Autodesk Inventor part; units mm, degrees
ref_plane "YZ Plane" through (0, 0, 0) normal (1, 0, 0) x (0, 1, 0)
ref_plane "XZ Plane" through (0, 0, 0) normal (0, 1, 0) x (-1, 0, 0)
ref_plane "XY Plane" through (0, 0, 0) normal (0, 0, 1) x (1, 0, 0)
sketch "Эскиз1" plane through (0, 0, 0) normal (0, 1, 0) x (-1, 0, 0)
  line L0 (-150, 150) -> (150, 150)
  line L1 (150, 150) -> (150, -150)
  line L2 (150, -150) -> (-150, -150)
  line L3 (-150, -150) -> (-150, 150)
  line L4 (-150, 150) -> (150, -150) construction
  line L5 (150, 150) -> (-150, -150) construction
  circle A0 centre (125, -125) radius 8.5
  circle A1 centre (0, -125) radius 8.5
  circle A2 centre (-125, -125) radius 8.5
  circle A3 centre (125, 125) radius 8.5
  circle A4 centre (0, 125) radius 8.5
  circle A5 centre (40, 100) radius 8.5
  circle A6 centre (40, 65) radius 8.5
  circle A7 centre (40, 30) radius 8.5
  circle A8 centre (-40, 30) radius 8.5
  circle A9 centre (-40, 65) radius 8.5
  circle A10 centre (-40, 100) radius 8.5
  circle A11 centre (-125, -125) radius 8.5
  circle A12 centre (-125, 125) radius 8.5
  point P0 (0, 0)
  point P1 (0, 0)
  point P2 (0, 0)
  dimension "d0" = 300
  dimension "d1" = 300
  dimension "d2" = 17
  dimension "d3" = 50
  dimension "d4" = 85
  dimension "d5" = 120
  dimension "d6" = 80
  dimension "d7" = 40
  dimension "d8" = 25
  dimension "d9" = 25
  dimension "d10" = 25
  dimension "d11" = 25
extrude "Пластина1" add sketch "Эскиз1" along normal blind 15
equation "\"d12\" = Толщина"
equation "\"Радиус_гибки\" = Толщина"
equation "\"Ширина_просечки\" = Толщина"
equation "\"Глубина_просечки\" = 0.5 * Толщина"
equation "\"Радиус_перехода\" = Радиус_гибки"
equation "\"Радиус_Якоби\" = Радиус_гибки"
equation "\"Размер_зазора\" = Толщина"
properties part number "Lift.00.00.00.01"
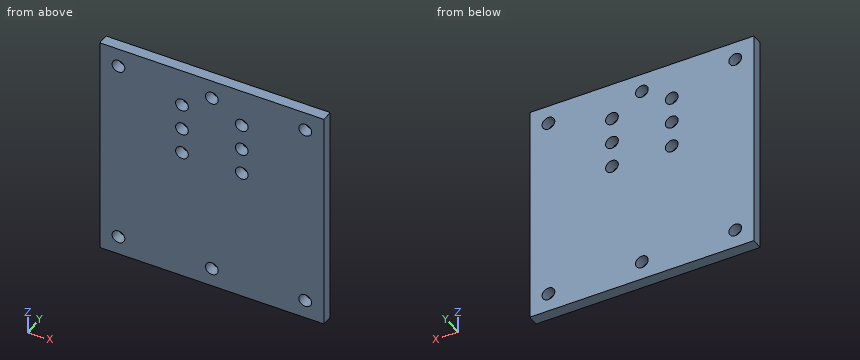
CAD build for the part. Positions are in the model's coordinates, mm. Coordinates: 2 decimals unless noted, no trailing zeros. Order: outer loops, then holes, each group sorted by start corner. A loop starts at its lowest first (then second) coordinate and runs counter-clockwise, first axis right, second up. Notation, with made-up numbers: (-17.5, 53.5) -> (-6.5, 53.5) arc R28 ccw to (-6.5, 81.5) -> close; hole circle Ø11 at (-8, 2). An arc over 180 degrees is marked (long way). Answer in a Markdown table with one row per item.
1) Band-saw the part on A-A (z = -125). List the corners of the cut face in (x, y), and give its area (4 significant figures).
Check values:
| item | result |
|---|---|
| outline | (-150, 0) -> (-133.5, 0) -> (-133.5, 15) -> (-150, 15) -> close; (-116.5, 0) -> (-8.5, 0) -> (-8.5, 15) -> (-116.5, 15) -> close; (8.5, 0) -> (116.5, 0) -> (116.5, 15) -> (8.5, 15) -> close; (133.5, 0) -> (150, 0) -> (150, 15) -> (133.5, 15) -> close |
| area | 3,735 mm2 |
2) Band-saw the part on C-C (x = 0). List the corners of the cut face in (y, z).
Check values:
| item | result |
|---|---|
| outline | (0, -150) -> (15, -150) -> (15, -133.5) -> (0, -133.5) -> close; (0, -116.5) -> (15, -116.5) -> (15, 116.5) -> (0, 116.5) -> close; (0, 133.5) -> (15, 133.5) -> (15, 150) -> (0, 150) -> close |
3) Flat gauge pin, fed straight in: P1, Ø22, axis at x = -40, z = 30, coming from the +Y side. Where does the tip first touch, or does it go through?
Check values:
| item | result |
|---|---|
| P1 | y = 15 |
4) Drill centre lines: line 1 (Z direction, x = 0, y = 4.25); line 2 (Z direction, x = 33, y = 7.5); line 3 (X direction, y = 11, z = 127.5). Where is each one in solid material? Low to high.
Check values:
| item | result |
|---|---|
| line 1 | -150 to -133.5, -116.5 to 116.5, 133.5 to 150 |
| line 2 | -150 to 25.18, 34.82 to 60.18, 69.82 to 95.18, 104.82 to 150 |
| line 3 | -150 to -133.12, -116.88 to -8.12, 8.12 to 116.88, 133.12 to 150 |
5) Band-saw the part on B-B (y = 3.75). Give the number of separate pieces and of enclosed holes in the cut face, and give its area (3 significant figures).
Check values:
| item | result |
|---|---|
| separate pieces | 1 |
| enclosed holes | 12 |
| area | 87,300 mm2 |
6) Band-saw the part on D-D (z = 65). List the corners of the cut face in (x, y).
Check values:
| item | result |
|---|---|
| outline | (-150, 0) -> (-48.5, 0) -> (-48.5, 15) -> (-150, 15) -> close; (-31.5, 0) -> (31.5, 0) -> (31.5, 15) -> (-31.5, 15) -> close; (48.5, 0) -> (150, 0) -> (150, 15) -> (48.5, 15) -> close |
